Check sheet for the modelled part. Datum: model origin and axes. Units: mm. A direction names the side the tool comes from. Give positions to 0.01 mm unless a question says otherwise; leave off trailing zeros. Loops run counter-clockwise (first coordinate to the right, second up) from the corner with the lowest first, then second, coordinate; pieces in that order, holes last. Notation, with made-up numbers: (-1, 33.5) - (37, 33.5) arc R16 ccw to (37, 57.5) - close; hole circle Ø11 at (81.5, 60). An arc over 180 degrees is marked (long way). Answer in a Markdown table with one row per item. Add a question column.
(1) Sectioned sample at A-A on y = -110. Enter the section's corners in (x, z), then the cut area to 3 significant figures.
(2) Sectioned sample at C-C on x = 0. Enter the section's corners in (y, z).
(3) Thickness scan on L1, parallel to X at y = 36, z = 0.4; L2, parallel to X at y = -24, z = 2.9; L3, parallel to X at y = -61, z = 1.25. Record the ranges inside material, lowest first.
(4) Draft check along Y on faces 3 (the face through (-14.39, -89.63, 1.97)), 4 (the face through (22.39, 132.15, 1.97)), 5 (the face through (0, 2, 0)). Enter one of: released by +Y, released by -Y, zero draft, split by the parting line, or undercut.
(5) Sectioned sample at B-B on z = 2.8. Enter the section's corners in (x, y).
(6) Set-up check for faces 1 (the face through (22.55, -131.99, 1.97)), 2 (the face through (14.55, 89.47, 1.97)): record each of +Z, -Z, +X, -X, +Y, -Y from which the full face is reachable in a straight line by a thin tool's end or side.
(7) Sectioned sample at D-D on y = 3.5. Enter the section's corners in (x, z).
from build123d import *

# Parameters (mm, degrees)
SKETCH1_R           = 3.05
BOSS_EXTRUDE1_DEPTH = 4


with BuildPart() as part:
    # Sketch1 → Boss-Extrude1 (new body)
    with BuildSketch(Plane.XY):
        with BuildLine():
            Line((15.4, -135), (-15.4, -135))
            ThreePointArc((-15.4, -135), (-22.471067812, -132.071067812), (-25.4, -125))
            Line((-25.4, -125), (-25.4, 125))
            ThreePointArc((-25.4, 125), (-22.471067812, 132.071067812), (-15.4, 135))
            Line((-15.4, 135), (15.4, 135))
            ThreePointArc((15.4, 135), (22.471067812, 132.071067812), (25.4, 125))
            Line((25.4, 125), (25.4, -125))
            ThreePointArc((25.4, -125), (22.471067812, -132.071067812), (15.4, -135))
        make_face()
        with Locations((0, 110)):
            Circle(SKETCH1_R, mode=Mode.SUBTRACT)
        with Locations((0, -110)):
            Circle(SKETCH1_R, mode=Mode.SUBTRACT)
        with BuildLine():
            Line((-13.434486763, 57.416947085), (14.322530577, -90.110507285))
            ThreePointArc((14.322530577, -90.110507285), (13.896435307, -91.757104812), (12.357017341, -92.480314961))
            Line((12.357017341, -92.480314961), (-7.4, -92.480314961))
            ThreePointArc((-7.4, -92.480314961), (-14.471067812, -89.551382772), (-17.4, -82.480314961))
            Line((-17.4, -82.480314961), (-17.4, 57.047139409))
            ThreePointArc((-17.4, 57.047139409), (-15.585706121, 59.038499055), (-13.434486763, 57.416947085))
        make_face(mode=Mode.SUBTRACT)
        with BuildLine():
            Line((17.4, -44.459157406), (17.4, 82.480314961))
            ThreePointArc((17.4, 82.480314961), (14.471067812, 89.551382772), (7.4, 92.480314961))
            Line((7.4, 92.480314961), (-9.988611838, 92.480314961))
            ThreePointArc((-9.988611838, 92.480314961), (-11.528029804, 91.757104812), (-11.954125074, 90.110507285))
            Line((-11.954125074, 90.110507285), (13.434486763, -44.828965081))
            ThreePointArc((13.434486763, -44.828965081), (15.585706121, -46.450517051), (17.4, -44.459157406))
        make_face(mode=Mode.SUBTRACT)
    extrude(amount=BOSS_EXTRUDE1_DEPTH)


solid = part.part
Reply:
| question | item | result |
|---|---|---|
| 1 | outline | (-25.4, 0) - (-3.05, 0) - (-3.05, 4) - (-25.4, 4) - close; (3.05, 0) - (25.4, 0) - (25.4, 4) - (3.05, 4) - close |
| 1 | area | 179 mm^2 |
| 2 | outline | (-135, 0) - (-113.05, 0) - (-113.05, 4) - (-135, 4) - close; (-106.95, 0) - (-92.48, 0) - (-92.48, 4) - (-106.95, 4) - close; (-13.99, 0) - (26.57, 0) - (26.57, 4) - (-13.99, 4) - close; (92.48, 0) - (106.95, 0) - (106.95, 4) - (92.48, 4) - close; (113.05, 0) - (135, 0) - (135, 4) - (113.05, 4) - close |
| 3 | L1 | -25.4 to -17.4, -9.4 to -1.77, 17.4 to 25.4 |
| 3 | L2 | -25.4 to -17.4, 1.88 to 9.52, 17.4 to 25.4 |
| 3 | L3 | -25.4 to -17.4, 8.85 to 25.4 |
| 4 | face 3 | undercut |
| 4 | face 4 | released by +Y |
| 4 | face 5 | zero draft |
| 5 | outline | (-25.4, -125) arc R10 ccw to (-15.4, -135) - (15.4, -135) arc R10 ccw to (25.4, -125) - (25.4, 125) arc R10 ccw to (15.4, 135) - (-15.4, 135) arc R10 ccw to (-25.4, 125) - close; hole (-17.4, -82.48) arc R10 ccw to (-7.4, -92.48) - (12.36, -92.48) arc R2 ccw to (14.32, -90.11) - (-13.43, 57.42) arc R2 ccw to (-17.4, 57.05) - close; hole (-11.95, 90.11) - (13.43, -44.83) arc R2 ccw to (17.4, -44.46) - (17.4, 82.48) arc R10 ccw to (7.4, 92.48) - (-9.99, 92.48) arc R2 ccw to start; hole circle Ø6.1 at (0, -110); hole circle Ø6.1 at (0, 110) |
| 6 | face 1 | +Z, -Z, +X, -Y |
| 6 | face 2 | +Z, -Z |
| 7 | outline | (-25.4, 0) - (-17.4, 0) - (-17.4, 4) - (-25.4, 4) - close; (-3.29, 0) - (4.34, 0) - (4.34, 4) - (-3.29, 4) - close; (17.4, 0) - (25.4, 0) - (25.4, 4) - (17.4, 4) - close |
